Input: part model. Units: mm. Frame: model coordinates. A direction names the side the tool comes from. Give positions to 0.01 mm unless a question says otherwise; leave off trailing zeros. Loops run counter-clockwise (first coordinate to the right, second up) from the corner with the lowest first, then second, coordinate; pieces in that order, holes last. Notation, with made-up numbers: (27.25, 57.5) - (42.25, 57.5) arc R8 cw to (42.25, 72.5) - close; hole circle Ø2 at (58, -8). An arc over 180 degrees is marked (long way). Answer as a JSON object with one key per item and string values.
from build123d import *

# Parameters (mm, degrees)
F2_W     = 29.6725835651
F2_H     = 153.1317234039
F3_DEPTH = 41.148


# Not quite as in the source:
# - the program builds the solid bodies; features that only make, move or delete a surface that nothing else refers to are left out


with BuildPart() as f1:
    # F0 (on Front) → F1 (revolve)
    with BuildSketch(Plane.XZ):
        Polygon((0, 42.5218716264), (0, -38.5478623211), (44.3764105439, -29.5401159674), (73.7840533257, -11.5246195346), align=None)
    revolve(axis=Axis((0, 0, 1.9870046526), (0, 0, -1)))

    # F2 (on Top) → F3 (join)
    with BuildSketch(Plane.XY):
        with Locations((-38.5478632525, 0.6623342633)):
            Rectangle(F2_W, F2_H)
        with Locations((38.5478632525, 0.6623342633)):
            Rectangle(F2_W, F2_H)
    extrude(amount=-F3_DEPTH)


solid = f1.part
Item 1: Cut plane A-A (z = 36). Return loops of the section in (x, y).
Geometry check:
{"outline": "circle Ø17.81 at (0, 0)"}
Item 2: Mould query, pull axis X, two halves, no side actions, for faces 6 (the face through (-53.384, 0, -25)), 7 (the face through (-42, -61, 0)), 8 (the face through (2.648, -0.834, -37.984)), 9 (the face through (61.46, 0.66, -19.07)). Classes: released by +X, released by -X, zero draft, split by the parting line, or undercut.
Geometry check:
{"face 6": "released by -X", "face 7": "zero draft", "face 8": "undercut", "face 9": "released by +X"}
Item 3: Cut plane B-B (z = 2). Return loops of the section in (x, y).
Geometry check:
{"outline": "circle Ø110.64 at (0, 0)"}
Item 4: Contact query for flat-ended pins moving along their axis: P1, Ø12.5, axis at y = -35, z = -27.5, coming from the +X side; P2, Ø4, axis at x = -15.5, y = 4.5, coming from the -Z side; P3, Ø1, axis at y = -17.5, z = 9, coming from the -X side. Output: stop coordinate, or through.
Geometry check:
{"P1": "stops at x = 53.38", "P2": "stops at z = -35.68", "P3": "stops at x = -43.05"}
Item 5: Access query for faces 1 (the face through (42, 56, 0)), 2 (the face through (-39, 2, -41.148)), 3 (the face through (-42, 56, 0)), 4 (the face through (42, -61, 0)), 5 (the face through (5.44, 10.45, 33.89)). Directions: +Z, -Z, +X, -X, +Y, -Y. A direction counts if a zero-diameter tool reaches every point of the face in a straight line with its end or side. Return the directions, or none.
Geometry check:
{"face 1": "+Z, +X, +Y", "face 2": "-Z, +X, -X, +Y, -Y", "face 3": "+Z, -X, +Y", "face 4": "+Z, +X, -Y", "face 5": "+Z"}
Item 6: Material intervals for line 1 (Z direction, x = 30.5, y = 56); line 2 (X direction, y = -54.5, z = -18); line 3 (Z direction, x = -32, y = -30), sorted ascending. Write a range as [from, to].
Geometry check:
{"line 1": "z = [-41.15, 0]", "line 2": "x = [-53.38, 53.38]", "line 3": "z = [-41.15, 10.39]"}
